```python
from build123d import *

# Parameters (mm, degrees)
F0_R     = 9.15
F1_DEPTH = 65
F4_R     = 1


with BuildPart() as f1:
    # F0 (on Top) → F1 (new body)
    with BuildSketch(Plane.XY):
        Circle(F0_R)
    extrude(amount=F1_DEPTH)

    # F2 (on Front) → F3 (revolve, cut)
    with BuildSketch(Plane.XZ):
        with BuildLine():
            Line((9.15, 4.25), (9.15, 5.75))
            ThreePointArc((9.15, 5.75), (8.4, 5), (9.15, 4.25))
        make_face()
    revolve(axis=Axis((0, 0, 13.149248), (0, 0, 1)), mode=Mode.SUBTRACT)

    # F4
    f4_edges = [f1.edges().sort_by_distance(p)[0] for p in [
        (-9.15, 0, 65),
        (-9.15, 0, 0),
    ]]
    fillet(f4_edges, radius=F4_R)


solid = f1.part
```
Source: CAD feature listing. Evaluate the final solid. Frame: model axes, mm. Round coordinates to 2 decimals unless told otherwise and drop trailing zeros. Order: outer loops, then holes, each group sorted by start corner. A loop starts at its lowest first (then second) coordinate and runs counter-clockwise, first axis right, second up. Notation, with made-up numbers: (84, -4.75) -> (94, -4.75) arc R31 ccw to (94, 27.25) -> close; hole circle Ø1 at (47, 4.25). An arc over 180 degrees is marked (long way). One line per item, written item: value. Start each with the question number.
Q1. Material intervals for probe 1 along X at (y, z) = (-0.5, 42.5); probe 2 along Z at (x, y) = (7.5, 5); probe 3 along Y at (x, z) = (-0.25, 23), sorted ascending.
Q2. Section query A-A (z = 51.5). Return the cut outline in (x, y).
Q3. Pin query (flat end, axial travel): pin 1 (5 mm diameter, centred on x = -7.5, z = 17, fed in from -Y); pin 2 (1.5 mm diameter, centred on x = -7, z = 13.5, fed in from +Y). Return the tip coordinate at first contact, or that it passes through.
Findings below:
1. probe 1: -9.14 to 9.14
1. probe 2: 0.5 to 4.26, 5.74 to 64.5
1. probe 3: -9.15 to 9.15
2. outline: circle Ø18.3 at (0, 0)
3. pin 1: y = -7.66
3. pin 2: y = 6.68
